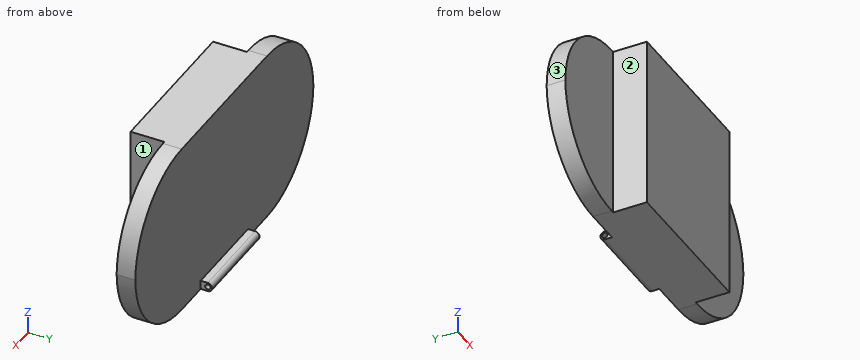
from build123d import *

# Parameters (mm, degrees)
SKETCH1_W           = 380
SKETCH1_H           = 195
BOSS_EXTRUDE1_DEPTH = 59
SKETCH2_W           = 195
SKETCH2_H           = 38
CUT_EXTRUDE1_DEPTH  = 102
FILLET1_R           = 99
SKETCH3_W           = 101
SKETCH3_H           = 10
BOSS_EXTRUDE2_DEPTH = 13
FILLET2_R           = 5
SKETCH4_R           = 3
CUT_EXTRUDE2_DEPTH  = 112


# Some blends are built 0.0001 mm under size
with BuildPart() as part:
    # Sketch1 → Boss-Extrude1 (new body)
    with BuildSketch(Plane(origin=(0, 0, 0), x_dir=(1, 0, 0), z_dir=(0, 1, 0))):
        Rectangle(SKETCH1_W, SKETCH1_H)
    extrude(amount=BOSS_EXTRUDE1_DEPTH)

    # Sketch2 → Cut-Extrude1 (cut)
    with BuildSketch(Plane(origin=(190, 0, 0), x_dir=(0, 0, -1), z_dir=(1, 0, 0))):
        with Locations((0, 19)):
            Rectangle(SKETCH2_W, SKETCH2_H)
    cut_extrude1 = extrude(amount=-CUT_EXTRUDE1_DEPTH, mode=Mode.SUBTRACT)

    # Mirror1: Cut-Extrude1 across plane
    add(cut_extrude1.mirror(Plane(origin=(0, 0, 0), x_dir=(0, 0, 1), z_dir=(1, 0, 0))), mode=Mode.SUBTRACT)

    # Fillet1
    # the kernel refuses this fillet: 99 mm, written as the material it takes off along each edge
    with BuildSketch(Plane(origin=(-190, -209.5, 97.5), x_dir=(0, 0, -1), z_dir=(0, 1, 0)), Plane(origin=(-190, -209.5, -97.5), x_dir=(1, 0, 0), z_dir=(0, 1, 0))) as fillet1_piece_1:
        with BuildLine():
            CenterArc((FILLET1_R, -FILLET1_R), FILLET1_R, 90, 90)
            Line((0, -FILLET1_R), (0, 0))
            Line((0, 0), (FILLET1_R, 0))
        make_face()
    extrude(amount=516, mode=Mode.SUBTRACT)
    with BuildSketch(Plane(origin=(190, -209.5, -97.5), x_dir=(-1, 0, 0), z_dir=(0, 1, 0)), Plane(origin=(190, -209.5, 97.5), x_dir=(0, 0, -1), z_dir=(0, 1, 0))) as fillet1_piece_2:
        with BuildLine():
            CenterArc((FILLET1_R, FILLET1_R), FILLET1_R, 180, 90)
            Line((0, FILLET1_R), (0, 0))
            Line((0, 0), (FILLET1_R, 0))
        make_face()
    extrude(amount=516, mode=Mode.SUBTRACT)

    # Sketch3 → Boss-Extrude2 (add)
    with BuildSketch(Plane(origin=(0, 59, 0), x_dir=(1, 0, 0), z_dir=(0, 1, 0))):
        with Locations((0, 92.5)):
            Rectangle(SKETCH3_W, SKETCH3_H)
    extrude(amount=BOSS_EXTRUDE2_DEPTH)

    # Fillet2
    fillet2_edges = [part.edges().sort_by_distance(p)[0] for p in [
        (0, 72, -97.5),
        (0, 72, -87.5),
    ]]
    fillet(fillet2_edges, radius=FILLET2_R - 0.0001)  # a hair under: the kernel refuses the full size

    # Sketch4 → Cut-Extrude2 (cut)
    with BuildSketch(Plane.ZY.offset(50.5)):
        with Locations((-92.5, 67)):
            Circle(SKETCH4_R)
    extrude(amount=-CUT_EXTRUDE2_DEPTH, mode=Mode.SUBTRACT)


solid = part.part
Input: part model. Units: mm. Frame: model coordinates. Face numbers are marked on the shaded views. A direction names the side the tool comes from. Round coordinates to 2 decimals unless told otherwise and drop trailing zeros. Write each loop counter-clockwise with the first axis right and the second up, starting at its lowest first coordinate (ties: lowest second). Pieces come first, ordered by that corner, then holes.
1) Ray query, L1, parallel to Y at x = -14.5, z = -92.5; L2, parallel to X at y = 34.5, z = 1; L3, parallel to Y at x = 90, z = 31.5. Return the intervals inside material, ascending.
2) Reachability of the marked faces 1, 2 and 3 from +Z, -Z, +X, -X, +Y, -Y: full face, straight path, thin tool, end or side. Return the list, or none.
3) Cut plane B-B (z = -25). Return the cut outline in (x, y), then the cut area to 3 significant figures.
4) Cut plane D-D (z = -74). Return the cut outline in (x, y), then the cut area to 3 significant figures.
5) Cut plane A-A (y = 43). Return the cut outline in (x, z).
6) Cut plane C-C (x = -76). Return the cut outline in (y, z), then the cut area to 3 significant figures.
7) Contact query for flat-ended pins moving along their axis: P1, Ø3, axis at y = 62.5, z = -93, coming from the -X side; P2, Ø5, axis at x = -112, y = 56.5, coming from the -Z side; P3, Ø5, axis at y = 68.5, z = -94, coming from the +X side; P4, Ø3.5, axis at y = 67, z = -92.5, coming from the -X side. Output: stop coordinate, or through.
Geometry says:
1. L1: y = 0 to 64, 70 to 72
1. L2: x = -88 to 88
1. L3: y = 38 to 59
2. face 1: +Z, -Z, +X, -Y
2. face 2: +Z, -Z, -X, -Y
2. face 3: +Z, -X, +Y, -Y
3. outline: (-186.39, 38) - (-88, 38) - (-88, 0) - (88, 0) - (88, 38) - (186.39, 38) - (186.39, 59) - (-186.39, 59) - close
3. area: 14,500 mm2
4. outline: (-155.04, 38) - (-88, 38) - (-88, 0) - (88, 0) - (88, 38) - (155.04, 38) - (155.04, 59) - (-155.04, 59) - close
4. area: 13,200 mm2
5. outline: (-189.99, 0) arc R99 ccw to (-91, -97.5) - (91, -97.5) arc R99 ccw to (189.99, 0) arc R99 ccw to (91, 97.5) - (-91, 97.5) arc R99 ccw to start
6. outline: (0, -97.5) - (59, -97.5) - (59, 97.5) - (0, 97.5) - close
6. area: 11,500 mm2
7. P1: stops at x = -50.5
7. P2: stops at z = -95.76
7. P3: stops at x = 50.5
7. P4: passes through
